Source: CAD feature listing. Evaluate the final solid. Frame: model axes, mm. A direction names the side the tool comes from. Give positions to 0.01 mm unless a question says otherwise; leave off trailing zeros. Order: outer loops, then holes, each group sorted by start corner. A loop starts at its lowest first (then second) coordinate and runs counter-clockwise, first axis right, second up.
Autodesk Inventor part; units mm, degrees
ref_plane "YZ Plane" through (0, 0, 0) normal (1, 0, 0) x (0, 1, 0)
ref_plane "XZ Plane" through (0, 0, 0) normal (0, 1, 0) x (-1, 0, 0)
ref_plane "XY Plane" through (0, 0, 0) normal (0, 0, 1) x (1, 0, 0)
sketch "Sketch1" plane through (0, 0, 0) normal (0, 0, 1) x (1, 0, 0)
  line L0 (0, 0) -> (30.25, 0) construction
  line L1 (0, 0) -> (-30.25, 0) construction
  line L2 (-30.25, 0) -> (-30.25, 40) construction
  line L3 (-30.25, 0) -> (-30.25, -40) construction
  circle A0 centre (-30.25, 40) radius 2.7
  circle A1 centre (-30.25, -40) radius 2.7
  circle A2 centre (30.25, 0) radius 2.7
  circle A3 centre (-30.25, 40) radius 12
  circle A4 centre (-30.25, -40) radius 12
  circle A5 centre (30.25, 0) radius 12
  line L4 (36.868172, -10.009985) -> (-23.631828, -50.009985)
  line L5 (-42.25, 40) -> (-42.25, -40)
  circle A6 centre (-34.25, 0) radius 2
  line L6 (-30.25, 0) -> (-34.25, 0) construction
  line L7 (-23.631828, 50.009985) -> (36.868172, 10.009985)
  line L8 (30.25, 0) -> (50.25, 0) construction
  circle A7 centre (50.25, 0) radius 10
  circle A8 centre (50.25, 0) radius 2
  line L9 (50.25746, 9.999997) -> (36.868172, 10.009985)
  line L10 (50.25746, -9.999997) -> (36.868172, -10.009985)
  circle A9 centre (10.25, 0) radius 2
  line L11 (50.25746, -9.999997) -> (60.257457, -9.992538)
  line L12 (60.257457, -9.992538) -> (60.242549, 9.992549)
  line L13 (60.242549, 9.992549) -> (50.25746, 9.999997)
  point P0 (-42.25, 0)
  point P1 (41.35, -4.559605)
  point P2 (41.35, 4.559605)
  point P3 (60.249997, 0.00746)
  dimension "d0" = 60.5
  dimension "d1" = 5.4
  dimension "d2" = 80
  dimension "d3" = 24
  dimension "d55" = 4
  dimension "d56" = 8
  dimension "d57" = 20
  dimension "d58" = 20
  dimension "d69" = 20
sketch "Sketch1 outline for Extrusion1" plane through (0, 0, 0) normal (0, 0, 1) x (1, 0, 0)
  arc A0 (-23.631828, 50.009985) -> (-42.25, 40) centre (-30.25, 40) ccw
  line L0 (-42.25, 40) -> (-42.25, -40)
  arc A1 (-42.25, -40) -> (-23.631828, -50.009985) centre (-30.25, -40) ccw
  line L1 (-23.631828, -50.009985) -> (36.868172, -10.009985)
  line L2 (36.868172, -10.009985) -> (60.257457, -9.992538)
  line L3 (60.257457, -9.992538) -> (60.242549, 9.992549)
  line L4 (60.242549, 9.992549) -> (36.868172, 10.009985)
  line L5 (36.868172, 10.009985) -> (-23.631828, 50.009985)
  circle A2 centre (-30.25, 40) radius 2.7
  circle A3 centre (10.25, 0) radius 2
  circle A4 centre (-34.25, 0) radius 2
  circle A5 centre (30.25, 0) radius 2.7
  circle A6 centre (-30.25, -40) radius 2.7
  circle A7 centre (50.25, 0) radius 2
extrude "Extrusion1" add sketch "Sketch1 outline for Extrusion1" against normal blind 10
fillet "Fillet1" radius 20 2 edges at (36.8682, 10.01, -5) (36.8682, -10.01, -5)
sketch "Sketch5" plane through (0, 0, 0) normal (0, 0, 1) x (1, 0, 0)
  arc A0 (-42.25, -40) -> (-23.631828, -50.009985) centre (-30.25, -40) ccw
  line L0 (-23.631828, -50.009985) -> (31.85846, -13.322191)
  arc A1 (42.873828, -10.005505) -> (31.85846, -13.322191) centre (42.888747, -30.0055) ccw
  line L1 (42.873828, -10.005505) -> (60.257457, -9.992538)
  arc A2 (31.85846, 13.322191) -> (42.873828, 10.005505) centre (42.888747, 30.0055) ccw
  line L2 (31.85846, 13.322191) -> (-23.631828, 50.009985)
  arc A3 (-23.631828, 50.009985) -> (-42.25, 40) centre (-30.25, 40) ccw
  line L3 (-42.25, 40) -> (-42.25, -40)
  circle A4 centre (-30.25, -40) radius 2.7
  circle A5 centre (30.25, 0) radius 2.7
  circle A6 centre (-34.25, 0) radius 2
  circle A7 centre (-30.25, 40) radius 2.7
  circle A8 centre (50.25, 0) radius 2
  line L4 (-4.75, 10) -> (-4.75, 37.526132)
  line L5 (-4.75, 10) -> (25.25, 10)
  line L6 (25.25, 10) -> (25.25, 17.691421)
  line L7 (60.257457, -9.992538) -> (60.242549, 9.992549)
  line L8 (60.242549, 9.992549) -> (42.873828, 10.005505)
  point P0 (10.267224, 24.242705)
  point P1 (8.658764, 37.564896)
  dimension "d64" = 10
  dimension "d65" = 5
  dimension "d66" = 30
extrude "Extrusion6" add sketch "Sketch5" along normal blind 20 contours L2 L6 L5 L4
sketch "Sketch6" plane through (-4.75, 10, 0) normal (0, -1, 0) x (1, 0, 0)
  line L0 (30, 0) -> (30, 20)
  line L1 (0, 20) -> (30, 20)
  line L2 (0, 0) -> (0, 20)
  line L3 (13, 0) -> (17, 0)
  line L4 (15, 0) -> (15, 10) construction
  circle A0 centre (15, 10) radius 2
  point P0 (4.75, 0)
  dimension "d70" = 10
  dimension "d71" = 4
ref_plane "Work Plane1" through (-4.75, 13, 0) normal (0, -1, 0) x (1, 0, 0)
extrude "Extrusion7" cut sketch "Sketch6" against normal through all
sketch "Sketch7" plane through (-4.75, 13, 0) normal (0, -1, 0) x (1, 0, 0)
  circle A0 centre (15, 10) radius 2
  circle A1 centre (15, 10) radius 4.5
  point P0 (4.75, 0)
  dimension "d75" = 9
extrude "Extrusion8" cut sketch "Sketch7" against normal through all
chamfer "Chamfer6" distance 2 angle 45 2 edges at (60.2425, 9.9925, -5) (60.2575, -9.9925, -5)
equation "\"b\" = 2"
properties part number "y axis something back_3DPrint"
1) Ray query, L1, parallel to Z at x = 10.25, y = 11.3; L2, parallel to Z at x = 10.25, y = 23; L3, parallel to Y at x = 50.25, z = -6.75. Return the intervals inside material, ascending.
Checks:
L1: z = -10 to 8, 12 to 20
L2: z = -10 to 5.5, 14.5 to 20
L3: y = -10 to -2, 2 to 10
2) Pull-direction query (X, two-part tool) for faces 4 (the face through (-30.835, -42.636, -4.93)), 5 (the face through (10, 10, 7.6)), 6 (the face through (37.04, -10.88, -5.07)), 7 (the face through (-30.835, 37.364, -4.93)); classes: +X half, -X half, draft (parallel to the pull), parting line (faces both ways), or undercut.
Checks:
face 4: undercut
face 5: draft
face 6: +X half
face 7: undercut
3) Section query D-D on x = 50.25. Output: boundary loops of the cut face in (y, z).
Checks:
outline: (-10, -10) - (-2, -10) - (-2, 0) - (-10, 0) - close; (2, -10) - (10, -10) - (10, 0) - (2, 0) - close
4) First-contact query: pin 1 Ø16 at (y, z) = (28.5, 10.5) entering from -X; pin 2 Ø8.5 at (y, z) = (14, 8.5) entering from +X; pin 3 Ø16 at (x, z) = (15.5, 12.5) entering from -Y. Flat tips, straight axial feed; report the tip coordinate or a pass-through.
Checks:
pin 1: stops at x = -4.75
pin 2: stops at x = 25.25
pin 3: stops at y = 10
5) Section query A-A on x = -30.25. Output: boundary loops of the cut face in (y, z).
Checks:
outline: (-52, -10) - (-42.7, -10) - (-42.7, 0) - (-52, 0) - close; (-37.3, -10) - (37.3, -10) - (37.3, 0) - (-37.3, 0) - close; (42.7, -10) - (52, -10) - (52, 0) - (42.7, 0) - close
6) Reachability of faces 1 (the face through (25.25, 14, 10)), 2 (the face through (8.663, -1.217, -4.93)), 3 (the face through (5.754, 19.731, 10.198)) from +Z, -Z, +X, -X, +Y, -Y: full face, straight path, thin tool, end or side. Return the list, or none.
Checks:
face 1: +Z, +X, +Y, -Y
face 2: +Z, -Z
face 3: +Y
7) Section query B-B on z = -8. Output: boundary loops of the cut face in (x, y).
Checks:
outline: (-42.25, -40) arc R12 ccw to (-23.63, -50.01) - (31.86, -13.32) arc R20 cw to (42.87, -10.01) - (58.26, -9.99) - (60.26, -7.99) - (60.24, 7.99) - (58.24, 9.99) - (42.87, 10.01) arc R20 cw to (31.86, 13.32) - (-23.63, 50.01) arc R12 ccw to (-42.25, 40) - close; hole circle Ø4 at (-34.25, 0); hole circle Ø5.4 at (-30.25, -40); hole circle Ø5.4 at (-30.25, 40); hole circle Ø4 at (10.25, 0); hole circle Ø5.4 at (30.25, 0); hole circle Ø4 at (50.25, 0)
8) Section query C-C on y = 0. Output: boundary loops of the cut face in (x, z), and give its area (3 significant figures).
Checks:
outline: (-42.25, -10) - (-36.25, -10) - (-36.25, 0) - (-42.25, 0) - close; (-32.25, -10) - (8.25, -10) - (8.25, 0) - (-32.25, 0) - close; (12.25, -10) - (27.55, -10) - (27.55, 0) - (12.25, 0) - close; (32.95, -10) - (48.25, -10) - (48.25, 0) - (32.95, 0) - close; (52.25, -10) - (60.25, -10) - (60.25, 0) - (52.25, 0) - close
area: 851 mm2
